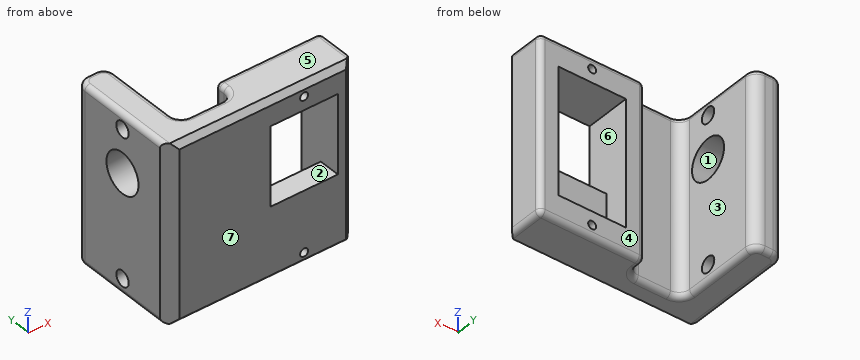
```python
from build123d import *

# Parameters (mm, degrees)
SKETCH048_W     = 21.6
SKETCH048_H     = 33
PAD018_DEPTH    = 5.5
SKETCH049_W     = 4.5
SKETCH049_H     = 33
PAD019_DEPTH    = 29.6
SKETCH050_W     = 33
SKETCH050_H     = 19.6
PAD020_DEPTH    = 4
SKETCH051_W     = 23.5
SKETCH051_H     = 12.6
POCKET023_DEPTH = 4.5
SKETCH052_W     = 14.7
SKETCH052_H     = 12.6
POCKET024_DEPTH = 4
SKETCH053_R     = 0.75
POCKET025_DEPTH = 9
CHAMFER007_SIZE = 1
CHAMFER008_SIZE = 2
FILLET010_R     = 2
FILLET013_R     = 2
FILLET014_R     = 2
FILLET015_R     = 1
FILLET016_R     = 1
SKETCH054_R     = 3.75
SKETCH054_R_2   = 1.45
POCKET026_DEPTH = 6


with BuildPart() as part:
    # Sketch048 → Pad018 (new body)
    with BuildSketch(Plane.YZ):
        with Locations((6.3, 0)):
            Rectangle(SKETCH048_W, SKETCH048_H)
    extrude(amount=PAD018_DEPTH)

    # Sketch049 (on Face6 of Pad018) → Pad019 (join)
    with BuildSketch(Plane.YZ.offset(5.5)):
        with Locations((-2.25, 0)):
            Rectangle(SKETCH049_W, SKETCH049_H)
    extrude(amount=PAD019_DEPTH)

    # Sketch050 (on Face9 of Pad019) → Pad020 (join)
    with BuildSketch(Plane.ZX):
        with Locations((0, 25.3)):
            Rectangle(SKETCH050_W, SKETCH050_H)
    extrude(amount=PAD020_DEPTH)

    # Sketch051 (on Face15 of Pad020) → Pocket023 (cut)
    with BuildSketch(Plane.ZX.offset(4)):
        with Locations((0, 25.3)):
            Rectangle(SKETCH051_W, SKETCH051_H)
    extrude(amount=-POCKET023_DEPTH, mode=Mode.SUBTRACT)

    # Sketch052 (on Face21 of Pocket023) → Pocket024 (cut)
    with BuildSketch(Plane.ZX.offset(-0.5)):
        with Locations((4.4, 25.3)):
            Rectangle(SKETCH052_W, SKETCH052_H)
    extrude(amount=-POCKET024_DEPTH, mode=Mode.SUBTRACT)

    # Sketch053 (on Face19 of Pocket024) → Pocket025 (cut)
    with BuildSketch(Plane.ZX.offset(4)):
        with Locations((-14.25, 25.3)):
            Circle(SKETCH053_R)
        with Locations((14.25, 25.3)):
            Circle(SKETCH053_R)
    extrude(amount=-POCKET025_DEPTH, mode=Mode.SUBTRACT)

    # Chamfer007
    chamfer007_edges = [part.edges().sort_by_distance(p)[0] for p in [
        (20.3, -4.5, 16.5),
        (20.3, -4.5, -16.5),
    ]]
    chamfer(chamfer007_edges, length=CHAMFER007_SIZE)

    # Chamfer008
    chamfer008_edges = [part.edges().sort_by_distance(p)[0] for p in [
        (0, -4.5, 0),
        (35.1, -4.5, 0),
    ]]
    chamfer(chamfer008_edges, length=CHAMFER008_SIZE)

    # Fillet010
    fillet010_edges = [part.edges().sort_by_distance(p)[0] for p in [
        (0, 17.1, 0),
        (5.5, 17.1, 0),
    ]]
    fillet(fillet010_edges, radius=FILLET010_R)

    # Fillet013
    fillet013_edges = [part.edges().sort_by_distance(p)[0] for p in [
        (5.5, 0, 0),
    ]]
    fillet(fillet013_edges, radius=FILLET013_R)

    # Fillet014
    fillet014_edges = [part.edges().sort_by_distance(p)[0] for p in [
        (15.5, 0, 0),
    ]]
    fillet(fillet014_edges, radius=FILLET014_R)

    # Fillet015
    fillet015_edges = [part.edges().sort_by_distance(p)[0] for p in [
        (15.5, 4, 0),
        (35.1, 4, 0),
    ]]
    fillet(fillet015_edges, radius=FILLET015_R)

    # Fillet016
    fillet016_edges = [part.edges().sort_by_distance(p)[0] for p in [
        (25.3, 4, 16.5),
        (25.3, 4, -16.5),
    ]]
    fillet(fillet016_edges, radius=FILLET016_R)

    # Sketch054 (on Face4 of Pocket025) → Pocket026 (cut)
    with BuildSketch(Plane(origin=(0, 0, 0), x_dir=(0, 1, 0), z_dir=(-1, 0, 0))):
        with Locations((6.3, -5.75)):
            Circle(SKETCH054_R)
        with Locations((6.3, -13.75)):
            Circle(SKETCH054_R_2)
        with Locations((6.3, 13.5)):
            Circle(SKETCH054_R_2)
    extrude(amount=-POCKET026_DEPTH, mode=Mode.SUBTRACT)


with BuildPart() as part_1:
    # Body005 placement: moved
    add(part.part.moved(Location((102, 0, 0))))


solid = part_1.part
```
The model under review builds one solid part; all positions refer to its coordinate system, in mm. Face numbers are marked on the shaded views. A direction names the side the tool comes from. Coordinates: 2 decimals unless noted, no trailing zeros. Order: outer loops, then holes, each group sorted by start corner. A loop starts at its lowest first (then second) coordinate and runs counter-clockwise, first axis right, second up. Notation, with made-up numbers: (58.5, 29) -> (83.5, 29) arc R19 cw to (83.5, 46) -> close; hole circle Ø2 at (4.5, 64). An arc over 180 degrees is marked (long way). Answer in a Markdown table with one row per item. Add a question column.
Item 1: Machinability: for the marked faces 1, 2, 3 and 4, which of the approach directions +Z, -Z, +X, -X, +Y, -Y give a long, thin tool a straight path to every point of the face, cutting with its end or side? Answer none if there is none.
Item 2: Mouldability with a two-part tool opening along Z and no side actions: class the marked faces 5, 6 and 7 as +Z half, -Z half, draft (parallel to the pull), parting line (faces both ways), or undercut.
Item 3: We need section A-A on x = 127.3. Write out the cut boundary in (y, z), plus the area to 3 significant figures.
Item 4: Clearance check with flat-ended pins moving along their axes: pin 1 (4 mm diameter, centred on x = 118, z = 11.5, fed in from +Y); pin 2 (3 mm diameter, centred on x = 115.5, z = -0.5, fed in from +Y); pin 3 (0.9 mm diameter, centred on x = 127.3, z = 14.25, fed in from -Y); pin 4 (6.5 mm diameter, centred on x = 112, z = -7.5, fed in from +Y). State where each tip first meets the part, or that it passes through.
Item 5: To check wall thickness, follow probe 1 along X at (y, z) = (2.5, 14.25); probe 2 along X at (y, z) = (2.25, 10); probe 3 along Z at (x, y) = (105.5, 6.3). State the ranges of each line that lie inside material, in increasing order.
Item 6: We need section D-D on z = -8. Write out the cut boundary in (x, y), plus the area to 3 significant figures.
Item 7: We need section B-B on y = 8.25. Write out the cut boundary in (x, z).
Item 8: We need section C-C on z = 9. Write out the cut boundary in (x, y).
Final values:
| question | item | result |
|---|---|---|
| 1 | face 1 | -X |
| 1 | face 2 | +Y, -Y |
| 1 | face 3 | +Z, -Z, +Y |
| 1 | face 4 | +Z, -Z, +X, +Y |
| 2 | face 5 | +Z half |
| 2 | face 6 | undercut |
| 2 | face 7 | draft |
| 3 | outline | (-4.5, -15.5) -> (-3.5, -16.5) -> (3, -16.5) arc R1 ccw to (4, -15.5) -> (4, -15) -> (-4.5, -15) -> close; (-4.5, -13.5) -> (4, -13.5) -> (4, -11.75) -> (-0.5, -11.75) -> (-0.5, -2.95) -> (-4.5, -2.95) -> close; (-4.5, 11.75) -> (4, 11.75) -> (4, 13.5) -> (-4.5, 13.5) -> close; (-4.5, 15) -> (4, 15) -> (4, 15.5) arc R1 ccw to (3, 16.5) -> (-3.5, 16.5) -> (-4.5, 15.5) -> close |
| 3 | area | 89.0 mm2 |
| 4 | pin 1 | stops at y = 4 |
| 4 | pin 2 | stops at y = 0.68 |
| 4 | pin 3 | passes through |
| 4 | pin 4 | stops at y = 0.15 |
| 5 | probe 1 | x = 102 to 107.5, 117.5 to 126.55, 128.05 to 137.1 |
| 5 | probe 2 | x = 102 to 107.5, 117.5 to 121, 133.6 to 137.1 |
| 5 | probe 3 | z = -16.5 to -14.95, -12.05 to 2, 9.5 to 12.3, 15.2 to 16.5 |
| 6 | outline | (102, -2.5) -> (104, -4.5) -> (135.1, -4.5) -> (137.1, -2.5) -> (137.1, 3) arc R1 ccw to (136.1, 4) -> (133.6, 4) -> (133.6, -0.5) -> (121, -0.5) -> (121, 4) -> (118.5, 4) arc R1 ccw to (117.5, 3) -> (117.5, 2) arc R2 cw to (115.5, 0) -> (109.5, 0) arc R2 cw to (107.5, 2) -> (107.5, 15.1) arc R2 ccw to (105.5, 17.1) -> (104, 17.1) arc R2 ccw to (102, 15.1) -> close |
| 6 | area | 269 mm2 |
| 7 | outline | (102, -15.5) arc R1 ccw to (103, -16.5) -> (106.5, -16.5) arc R1 ccw to (107.5, -15.5) -> (107.5, 2.55) -> (102, 2.55) -> close; (102, 8.95) -> (107.5, 8.95) -> (107.5, 15.5) arc R1 ccw to (106.5, 16.5) -> (103, 16.5) arc R1 ccw to (102, 15.5) -> close |
| 8 | outline | (102, -2.5) -> (104, -4.5) -> (121, -4.5) -> (121, 4) -> (118.5, 4) arc R1 ccw to (117.5, 3) -> (117.5, 2) arc R2 cw to (115.5, 0) -> (109.5, 0) arc R2 cw to (107.5, 2) -> (107.5, 4.43) -> (102, 4.43) -> close; (102, 8.17) -> (107.5, 8.17) -> (107.5, 15.1) arc R2 ccw to (105.5, 17.1) -> (104, 17.1) arc R2 ccw to (102, 15.1) -> close; (133.6, -4.5) -> (135.1, -4.5) -> (137.1, -2.5) -> (137.1, 3) arc R1 ccw to (136.1, 4) -> (133.6, 4) -> close |
